The drawing under review shows one solid part. Ordinate dimensions are in mm from its lowest x, y, z. A direction names the side the tool comes from. Round coordinates to 2 decimals unless told otherwise and drop trailing zeros. Order: outer loops, then holes, each group sorted by start corner. A loop starts at its lowest first (then second) coordinate and runs counter-clockwise, first axis right, second up. Notation, with made-up numbers: (-18, 10.25) -> (13, 10.25) arc R20 ccw to (13, 20.25) -> close; hole circle Ø7 at (30.25, 24.25). An arc over 180 degrees is marked (long way). Return JSON: item names as keys, results as strings. Group by question number.
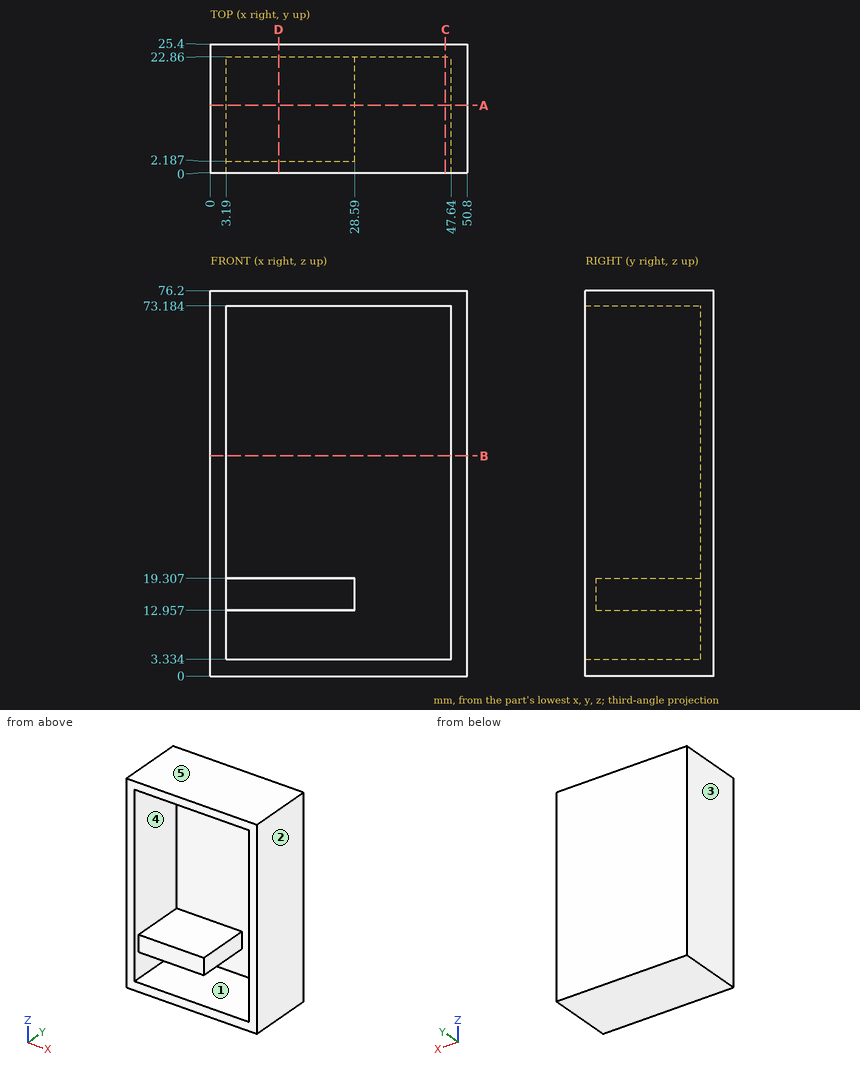
Item 1: Consider section D-D on x = 13.5. State the section outline as (y, z) points.
Item 2: The part is to be moulded in two halves that separate along Z. For the marked faces 3, 4 and 5, say which applies: +Z half, -Z half, draft (parallel to the pull), parting line (faces both ways), or undercut.
Item 3: Insertion check: pin 1 Ø6 at (x, z) = (8, 45) entering from -Y; pin 2 Ø3 at (x, z) = (12, 15) entering from -Y. Each pin has a flat end and moves straight along its axis. Give the tip position at first contact, or say it passes through.
Item 4: Consider section B-B on z = 43.5. State the section outline as (x, y) points, plus the area to 3 significant figures.
Item 5: For the marked faces 1 and 2, list the 3-axis set-ups (+Z, -Z, +X, -X, +Y, -Y) from which the entire face can be reached by the end or side of a thin tool; tool diameter is ignored.
Item 6: Wall thickness on line 1 along Z through (x, y) = (28, 15.5); line 2 along Z through (x, y) = (36, 17); line 3 along X through (y, z) = (14, 29): over which ranges is each line inside the solid? List them lowest first.
Item 7: Consider section C-C on x = 46.5. State the section outline as (y, z) points.
Item 8: Consider section A-A on y = 13.25. State the section outline as (x, z) points.
Values:
{
 "1": {"outline": "(0, 0) -> (25.4, 0) -> (25.4, 76.2) -> (0, 76.2) -> (0, 73.18) -> (22.86, 73.18) -> (22.86, 19.31) -> (2.19, 19.31) -> (2.19, 12.96) -> (22.86, 12.96) -> (22.86, 3.33) -> (0, 3.33) -> close"},
 "2": {"face 3": "draft", "face 4": "undercut", "face 5": "+Z half"},
 "3": {"pin 1": "y = 22.86", "pin 2": "y = 2.19"},
 "4": {"outline": "(0, 0) -> (3.19, 0) -> (3.19, 22.86) -> (47.64, 22.86) -> (47.64, 0) -> (50.8, 0) -> (50.8, 25.4) -> (0, 25.4) -> close", "area": "274 mm^2"},
 "5": {"face 1": "-Y", "face 2": "+Z, -Z, +X, +Y, -Y"},
 "6": {"line 1": "0 to 3.33, 12.96 to 19.31, 73.18 to 76.2", "line 2": "0 to 3.33, 73.18 to 76.2", "line 3": "0 to 3.19, 47.64 to 50.8"},
 "7": {"outline": "(0, 0) -> (25.4, 0) -> (25.4, 76.2) -> (0, 76.2) -> (0, 73.18) -> (22.86, 73.18) -> (22.86, 3.33) -> (0, 3.33) -> close"},
 "8": {"outline": "(0, 0) -> (50.8, 0) -> (50.8, 76.2) -> (0, 76.2) -> close; hole (3.19, 3.33) -> (47.64, 3.33) -> (47.64, 73.18) -> (3.19, 73.18) -> (3.19, 19.31) -> (28.59, 19.31) -> (28.59, 12.96) -> (3.19, 12.96) -> close"}
}
